Check sheet for the modelled part. Datum: model origin and axes. Units: mm. Face numbers are marked on the shaded views. A direction names the side the tool comes from. Give positions to 0.01 mm unless a question says otherwise; leave off trailing zeros. Answer as CSV lines item,"result". Start each with the question number.
(1) Release check for a two-part mould opening along Z. For the marked faces 3 and 4 record: pulls with the +Z half, pulls with the -Z half, needs draft (parallel to the pull), parting line crosses it, or undercut.
(2) Access from +Z, -Z, +X, -X, +Y, -Y to the whole of each face (thin tool, end or side, straight path). Record for the marked faces 1 and 2.
(3) Section check A-A on y = -2. State how many separate pieces and enclosed holes the cut face has, plus the area to 3 significant figures.
(4) Material ranges on line 1 (X direction, y = 5, z = 0) (3 decimals); line 2 (X direction, y = 11.5, z = 43), recorded low to high. Write a range as from..to.
(5) Gauge pin test, flat ends, axial feed: pin 1 Ø8.5 at (x, z) = (-25.51, 0) entering from -Y; pin 2 Ø5 at (x, z) = (-12.76, 22.09) entering from -Y; pin 3 Ø2 at (x, y) = (37.5, 21.5) entering from +Z; pin 4 Ø10 at (x, z) = (0.5, -24.5) entering from +Y. Record the tip position at first contact, or that the pin passes through.
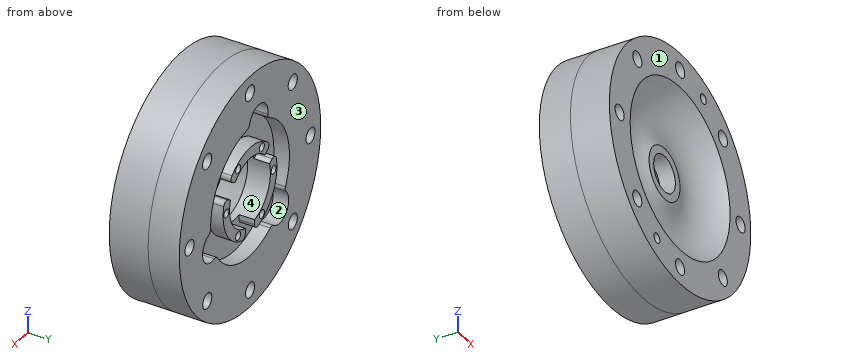
from build123d import *

# Parameters (mm, degrees)
SKETCH6_R                      = 42.5
SKETCH6_R_2                    = 29
CUT_EXTRUDE3_DEPTH             = 10
SKETCH7_W                      = 10
SKETCH7_H                      = 7.550043706
CUT_EXTRUDE4_DEPTH             = 10
CIRPATTERN2_COUNT              = 3
DELETEFACE1_START              = 15
DELETEFACE1_OUTLINE_R          = 76.2
DELETEFACE1_OUTLINE_R_2        = 55
DELETEFACE1_DEPTH              = 20
F_3_8_CLEARANCE_HOLE1_D        = 9.8044
SKETCH46_R                     = 10
CUT_EXTRUDE5_DEPTH             = 10
CIRPATTERN6_COUNT              = 3
FILLET2_R                      = 3
CIRPATTERN7_COUNT              = 6
F_1_4_0_2500_DOWEL_HOLE1_D     = 6.35
F_1_4_0_2500_DOWEL_HOLE1_DEPTH = 9.906
F_1_4_0_2500_DOWEL_HOLE1_TIP   = 1.907732465


# Read off the part's stored shape, not the designer's step: DeleteFace1
with BuildPart() as part:
    # Sketch3 → Revolve1 (revolve)
    with BuildSketch(Plane(origin=(0, 0, 0), x_dir=(0, 0, -1), z_dir=(1, 0, 0))):
        with BuildLine():
            Line((76.2, 15), (55, 15))
            Line((55, 15), (55, 35))
            Line((55, 35), (22.025, 35))
            Line((22.025, 35), (22.025, 20.36))
            Line((22.025, 20.36), (11.665, 10))
            Line((11.665, 10), (11.665, 0))
            Line((11.665, 0), (16.665, 0))
            ThreePointArc((16.665, 0), (37.471852779, 3.234070807), (53.85, -10))
            Line((53.85, -10), (76.2, -10))
            Line((76.2, -10), (76.2, 15))
        make_face()
    revolve(axis=Axis((0, 0, 0), (0, 1, 0)))

    # Sketch6 → Cut-Extrude3 (cut)
    with BuildSketch(Plane(origin=(0, 35, 0), x_dir=(1, 0, 0), z_dir=(0, 1, 0))):
        with Locations(Location((0, 0, 0), (0, 0, 270))):
            Circle(SKETCH6_R)
        with Locations(Location((0, 0, 0), (0, 0, 270))):
            Circle(SKETCH6_R_2, mode=Mode.SUBTRACT)
    extrude(amount=-CUT_EXTRUDE3_DEPTH, mode=Mode.SUBTRACT)

    # Sketch7 → Cut-Extrude4 (cut)
    with BuildSketch(Plane(origin=(0, 35, 0), x_dir=(1, 0, 0), z_dir=(0, 1, 0))):
        with Locations((0, 25.224978147)):
            Rectangle(SKETCH7_W, SKETCH7_H)
    cut_extrude4 = extrude(amount=-CUT_EXTRUDE4_DEPTH, mode=Mode.SUBTRACT)

    # CirPattern2: Cut-Extrude4 ×3 about axis
    cirpattern2_axis = Axis((0, 0, 0), (0, 1, 0))
    for i in range(1, CIRPATTERN2_COUNT):
        add(cut_extrude4.rotate(cirpattern2_axis, i * 360 / CIRPATTERN2_COUNT), mode=Mode.SUBTRACT)

    # DeleteFace1 outline → DeleteFace1 (add)
    with BuildSketch(Plane(origin=(0, 0, 0), x_dir=(1, 0, 0), z_dir=(0, 1, 0)).offset(DELETEFACE1_START)):
        Circle(DELETEFACE1_OUTLINE_R)
        Circle(DELETEFACE1_OUTLINE_R_2, mode=Mode.SUBTRACT)
    extrude(amount=DELETEFACE1_DEPTH)

    # 3/8 Clearance Hole1 (through all)
    with Locations(Plane(origin=(0, -10, 0), x_dir=(-1, 0, 0), z_dir=(0, -1, 0))):
        with Locations((46.153593538, 46.060907757), (65.203960939, -0.061814491), (46.060915247, -46.146148146), (-0.061807016, -65.196515566), (-46.146140681, -46.053469867), (-65.196508083, 0.069252405), (-46.053462365, 46.15358606), (0.069259897, 65.203953456)):
            Hole(F_3_8_CLEARANCE_HOLE1_D / 2)

    # Sketch46 → Cut-Extrude5 (cut)
    with BuildSketch(Plane(origin=(0, 35, 0), x_dir=(1, 0, 0), z_dir=(0, 1, 0))):
        with Locations((41.099239846, 12.958540547)):
            Circle(SKETCH46_R)
    cut_extrude5 = extrude(amount=-CUT_EXTRUDE5_DEPTH, mode=Mode.SUBTRACT)

    # CirPattern6: Cut-Extrude5 ×3 about axis
    cirpattern6_axis = Axis((0, 0, 0), (0, 1, 0))
    for i in range(1, CIRPATTERN6_COUNT):
        add(cut_extrude5.rotate(cirpattern6_axis, i * 360 / CIRPATTERN6_COUNT), mode=Mode.SUBTRACT)

    # Fillet2
    fillet2_edges = [part.edges().sort_by_distance(p)[0] for p in [
        (36.469652208, 30, -21.822338734),
        (42.390969445, 30, -3.042319763),
        (-37.133525818, 30, -20.672475912),
        (-23.830210924, 30, -35.190496549),
        (0.66387361, 30, 42.494814646),
        (-18.560758521, 30, 38.232816312),
        (5, 30, -28.565713714),
        (-5, 30, -28.565713714),
        (27.238633754, 30, 9.952729838),
        (22.238633754, 30, 18.612983876),
        (-22.238633754, 30, 18.612983876),
        (-27.238633754, 30, 9.952729838),
    ]]
    fillet(fillet2_edges, radius=FILLET2_R)

    # Sketch51 → 1/4-28 Tapped Hole1 (revolve, cut)
    with BuildSketch(Plane(origin=(25.5125, 35, 0), x_dir=(0, 0, 1), z_dir=(1, 0, 0))):
        Polygon((0, 0), (0, 17.045388061), (2.7051, 15.42), (2.7051, 0), align=None)
    f_1_4_28_tapped_hole1 = revolve(axis=Axis((25.5125, 41.35, 0), (0, -1, 0)), mode=Mode.SUBTRACT)

    # CirPattern7: 1/4-28 Tapped Hole1 ×6 about axis
    cirpattern7_axis = Axis((0, 0, 0), (0, 1, 0))
    for i in range(1, CIRPATTERN7_COUNT):
        add(f_1_4_28_tapped_hole1.rotate(cirpattern7_axis, i * 360 / CIRPATTERN7_COUNT), mode=Mode.SUBTRACT)

    # 1/4 (0.2500) Dowel Hole1
    with Locations(Plane(origin=(0, -10, 0), x_dir=(-1, 0, 0), z_dir=(0, -1, 0))):
        with Locations((-25.007850676, -60.207814752), (25.01513322, 60.21585851)):
            Hole(F_1_4_0_2500_DOWEL_HOLE1_D / 2, depth=F_1_4_0_2500_DOWEL_HOLE1_DEPTH)
            with Locations((0, 0, -(F_1_4_0_2500_DOWEL_HOLE1_DEPTH + F_1_4_0_2500_DOWEL_HOLE1_TIP / 2))):  # 118° drill point
                Cone(0, F_1_4_0_2500_DOWEL_HOLE1_D / 2, F_1_4_0_2500_DOWEL_HOLE1_TIP, mode=Mode.SUBTRACT)


solid = part.part
Working result:
1,face 3,"needs draft"
1,face 4,"undercut"
2,face 1,"+Z, -Z, +X, -X, -Y"
2,face 2,"+Y"
3,separate pieces,"1"
3,enclosed holes,"11"
3,area,"10,500 mm^2"
4,line 1,"x = -76.2..-70.106, -60.302..-11.665, 11.665..60.295, 70.098..76.2"
4,line 2,"x = -62.91..-49.82, -42.3..42.31, 49.98..62.91"
5,pin 1,"stops at y = 2.34"
5,pin 2,"stops at y = 2.96"
5,pin 3,"stops at z = 66.89"
5,pin 4,"stops at y = 35"
